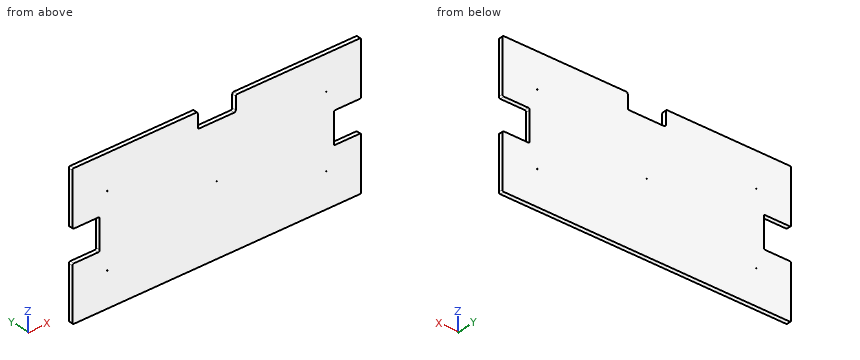
from build123d import *

# Parameters (mm, degrees)
SKETCH1_W                    = 1206.5
SKETCH1_H                    = 596.9
BOSS_EXTRUDE1_DEPTH          = 17.78
F_1_8_0_125_DIAMETER_HOLE1_D = 3.175
FILLET1_R                    = 6.35
SKETCH4_W                    = 158.75
SKETCH4_H                    = 66.04
SKETCH4_W_2                  = 114.3
SKETCH4_H_2                  = 133.35
CUT_EXTRUDE1_DEPTH           = 18.78
FILLET2_R                    = 6.35


with BuildPart() as part:
    # Sketch1 → Boss-Extrude1 (new body)
    with BuildSketch(Plane(origin=(0, 0, 0), x_dir=(1, 0, 0), z_dir=(0, 1, 0))):
        Rectangle(SKETCH1_W, SKETCH1_H)
    extrude(amount=BOSS_EXTRUDE1_DEPTH)

    # 1/8 (0.125) Diameter Hole1 (through all)
    with Locations(Plane(origin=(0, 17.78, 0), x_dir=(1, 0, 0), z_dir=(0, 1, 0))):
        with Locations((0, 0), (457.2, 152.4), (-457.2, -152.4), (-457.2, 152.4), (457.2, -152.4)):
            Hole(F_1_8_0_125_DIAMETER_HOLE1_D / 2)

    # Fillet1
    fillet1_edges = [part.edges().sort_by_distance(p)[0] for p in [
        (603.25, 8.89, 298.45),
        (-603.25, 8.89, 298.45),
        (-603.25, 8.89, -298.45),
        (603.25, 8.89, -298.45),
    ]]
    fillet(fillet1_edges, radius=FILLET1_R)

    # Sketch4 → Cut-Extrude1 (cut, through all)
    with BuildSketch(Plane(origin=(0, 17.78, 0), x_dir=(1, 0, 0), z_dir=(0, 1, 0))):
        with Locations((0, -265.43)):
            Rectangle(SKETCH4_W, SKETCH4_H)
        with Locations((-546.1, 0)):
            Rectangle(SKETCH4_W_2, SKETCH4_H_2)
        with Locations((546.1, 0)):
            Rectangle(SKETCH4_W_2, SKETCH4_H_2)
    extrude(amount=-CUT_EXTRUDE1_DEPTH, mode=Mode.SUBTRACT)

    # Fillet2
    fillet2_edges = [part.edges().sort_by_distance(p)[0] for p in [
        (-488.95, 8.89, 66.675),
        (603.25, 8.89, -66.675),
        (603.25, 8.89, 66.675),
        (488.95, 8.89, 66.675),
        (488.95, 8.89, -66.675),
        (79.375, 8.89, 232.41),
        (79.375, 8.89, 298.45),
        (-79.375, 8.89, 298.45),
        (-79.375, 8.89, 232.41),
        (-603.25, 8.89, 66.675),
        (-603.25, 8.89, -66.675),
        (-488.95, 8.89, -66.675),
    ]]
    fillet(fillet2_edges, radius=FILLET2_R)


solid = part.part
Input: part model. Units: mm. Frame: model coordinates. Coordinates: 2 decimals unless noted, no trailing zeros. Loops run counter-clockwise (first coordinate to the right, second up) from the corner with the lowest first, then second, coordinate; pieces in that order, holes last.
Q1. Material intervals for line 1 (Z direction, x = 457.2, y = 5.5); line 2 (X direction, y = 14, z = 152.4); line 3 (X direction, y = 4.75, z = 264) (3 decimals), sorted ascending.
Q2. Contact query for flat-ended pins moving along their axis: pin 1 (8 mm diameter, centred on y = 8, z = -2, fed in from +X); pin 2 (2.5 mm diameter, centred on x = 457.2, z = 152.4, fed in from -Y); pin 3 (1.5 mm diameter, centred on y = 14, z = -38.5, fed in from -X); pin 4 (5.5 mm diameter, centred on x = -11.5, y = 11.5, fed in from +Z). Output: stop coordinate, or through.
Q3. Cut plane B-B (z = -46). Output: boundary loops of the cut face in (x, y).
Q4. Cut plane A-A (y = 14.75). Give the number of separate pieces and of enclosed holes in the cut face, then the cut area to 3 significant figures.
Working result:
1. line 1: z = -298.45 to -153.99, -150.81 to 150.81, 153.99 to 298.45
1. line 2: x = -603.25 to -458.79, -455.61 to 455.61, 458.79 to 603.25
1. line 3: x = -603.25 to -79.375, 79.375 to 603.25
2. pin 1: stops at x = 488.95
2. pin 2: passes through
2. pin 3: stops at x = -488.95
2. pin 4: stops at z = 232.41
3. outline: (-488.95, 0) - (488.95, 0) - (488.95, 17.78) - (-488.95, 17.78) - close
4. separate pieces: 1
4. enclosed holes: 5
4. area: 679,000 mm2
